from build123d import *

# Parameters (mm, degrees)
BOSS_EXTRUDE1_DEPTH      = 8.2
BOSS_EXTRUDE1_DEPTH_BACK = 8.2
SKETCH2_W                = 10
SKETCH2_H                = 42
CUT_EXTRUDE1_DEPTH       = 25.662522174
CUT_EXTRUDE1_DEPTH_BACK  = 25.662522174
SKETCH4_R                = 1
SKETCH4_W                = 13.4
SKETCH4_H                = 24
CIRPATTERN1_COUNT        = 4
BOSS_EXTRUDE2_DEPTH      = 8
BOSS_EXTRUDE3_DEPTH      = 8
BOSS_EXTRUDE4_DEPTH      = 6
BOSS_EXTRUDE5_START      = 6
SKETCH23_R               = 37.2
BOSS_EXTRUDE5_DEPTH      = 6


with BuildPart() as part:
    # Sketch2 → Boss-Extrude1 (new, two sides: drawn at the far end of the back side and taken through both)
    with BuildSketch(Plane(origin=(0, 0, 0), x_dir=(0, 0, -1), z_dir=(1, 0, 0)).offset(-BOSS_EXTRUDE1_DEPTH_BACK)):
        with Locations((-22, 0)):
            Rectangle(SKETCH2_W, SKETCH2_H)
    extrude(amount=BOSS_EXTRUDE1_DEPTH + BOSS_EXTRUDE1_DEPTH_BACK)

    # Sketch4 → Cut-Extrude1 (cut, two sides: drawn at the far end of the back side and taken through both)
    with BuildSketch(Plane.XY.offset(27).offset(-CUT_EXTRUDE1_DEPTH_BACK)):
        with Locations((-3, 14.95)):
            Circle(SKETCH4_R)
        with Locations((2.95, 14.95)):
            Circle(SKETCH4_R)
        with Locations((-3, -14.95)):
            Circle(SKETCH4_R)
        with Locations((2.95, -14.95)):
            Circle(SKETCH4_R)
        with Locations((1.5, 0)):
            Rectangle(SKETCH4_W, SKETCH4_H)
    extrude(amount=CUT_EXTRUDE1_DEPTH + CUT_EXTRUDE1_DEPTH_BACK, mode=Mode.SUBTRACT)


with BuildPart() as cirpattern1_1:
    # CirPattern1: pattern copy
    add(part.part.rotate(Axis((0, 0, 0), (0, 1, 0)), 1 * 360 / CIRPATTERN1_COUNT))


with BuildPart() as cirpattern1_2:
    # CirPattern1: pattern copy
    add(part.part.rotate(Axis((0, 0, 0), (0, 1, 0)), 2 * 360 / CIRPATTERN1_COUNT))


with BuildPart() as cirpattern1_3:
    # CirPattern1: pattern copy
    add(part.part.rotate(Axis((0, 0, 0), (0, 1, 0)), 3 * 360 / CIRPATTERN1_COUNT))


with BuildPart() as part_1:
    add(part.part)

    add(cirpattern1_1.part)  # Boss-Extrude2 merges CirPattern1_1

    add(cirpattern1_2.part)  # Boss-Extrude2 merges CirPattern1_2

    add(cirpattern1_3.part)  # Boss-Extrude2 merges CirPattern1_3
    # Sketch20 → Boss-Extrude2 (add)
    with BuildSketch(Plane(origin=(0, 21, 0), x_dir=(1, 0, 0), z_dir=(0, 1, 0))):
        Polygon((-17, 8.2), (-8.2, 17), (-8.2, 27), (-27, 8.2), align=None)
        Polygon((-17, -8.2), (-8.2, -17), (-8.2, -27), (-27, -8.2), align=None)
        Polygon((8.2, -17), (17, -8.2), (27, -8.2), (8.2, -27), align=None)
        Polygon((8.2, 17), (17, 8.2), (27, 8.2), (8.2, 27), align=None)
    extrude(amount=-BOSS_EXTRUDE2_DEPTH)

    # Sketch21 → Boss-Extrude3 (add)
    with BuildSketch(Plane.XZ.offset(21)):
        Polygon((-17, 8.2), (-8.2, 17), (-8.2, 27), (-27, 8.2), align=None)
        Polygon((17, -8.2), (8.2, -17), (8.2, -27), (27, -8.2), align=None)
        Polygon((-8.2, -17), (-17, -8.2), (-27, -8.2), (-8.2, -27), align=None)
        Polygon((8.2, 17), (17, 8.2), (27, 8.2), (8.2, 27), align=None)
    extrude(amount=-BOSS_EXTRUDE3_DEPTH)

    # Sketch22 → Boss-Extrude4 (add)
    with BuildSketch(Plane.XZ.offset(21)):
        with BuildLine():
            ThreePointArc((-15.663157895, 33.741746913), (-26.30437226, 26.30437226), (-33.741746913, 15.663157895))
            Line((-33.741746913, 15.663157895), (-33.274371034, 15.663157895))
            Line((-33.274371034, 15.663157895), (-33.274371034, -15.663157895))
            Line((-33.274371034, -15.663157895), (-33.741746913, -15.663157895))
            ThreePointArc((-33.741746913, -15.663157895), (-26.30437226, -26.30437226), (-15.663157895, -33.741746913))
            Line((-15.663157895, -33.741746913), (-15.663157895, -33.274371034))
            Line((-15.663157895, -33.274371034), (15.663157895, -33.274371034))
            Line((15.663157895, -33.274371034), (15.663157895, -33.741746913))
            ThreePointArc((15.663157895, -33.741746913), (26.30437226, -26.30437226), (33.741746913, -15.663157895))
            Line((33.741746913, -15.663157895), (33.274371034, -15.663157895))
            Line((33.274371034, -15.663157895), (33.274371034, 15.663157895))
            Line((33.274371034, 15.663157895), (33.741746913, 15.663157895))
            ThreePointArc((33.741746913, 15.663157895), (26.30437226, 26.30437226), (15.663157895, 33.741746913))
            Line((15.663157895, 33.741746913), (15.663157895, 33.274371034))
            Line((15.663157895, 33.274371034), (-15.663157895, 33.274371034))
            Line((-15.663157895, 33.274371034), (-15.663157895, 33.741746913))
        make_face()
        Polygon((17, -8.2), (8.2, -17), (-8.2, -17), (-17, -8.2), (-17, 8.2), (-8.2, 17), (8.2, 17), (17, 8.2), align=None, mode=Mode.SUBTRACT)
    extrude(amount=BOSS_EXTRUDE4_DEPTH)

    # Sketch23 → Boss-Extrude5 (add)
    with BuildSketch(Plane(origin=(0, 21, 0), x_dir=(1, 0, 0), z_dir=(0, 1, 0)).offset(BOSS_EXTRUDE5_START)):
        with Locations(Location((0, 0, 0), (0, 0, 270))):
            Circle(SKETCH23_R)
        Polygon((-17, 8.2), (-8.2, 17), (8.2, 17), (17, 8.2), (17, -8.2), (8.2, -17), (-8.2, -17), (-17, -8.2), align=None, mode=Mode.SUBTRACT)
    extrude(amount=-BOSS_EXTRUDE5_DEPTH)


solid = part_1.part
Here's how the part is built. I have some questions about the finished solid (model axes, mm). A direction names the side the tool comes from. Give positions to 0.01 mm unless a question says otherwise; leave off trailing zeros. Order: outer loops, then holes, each group sorted by start corner. A loop starts at its lowest first (then second) coordinate and runs counter-clockwise, first axis right, second up. Notation, with made-up numbers: M 62.25,48.5 L 80.25,48.5 A21 cw 80.25,72.5 Z; hole C 19,-30.75 d11. An arc over 180 degrees is marked long. Answer as a JSON object with one key per item and string values. Group by question number.
1) Suppose I cut it at A-A, the plane y = 11. Write out the boundary of the cut face in (x, z), plus the area to 3 significant figures.
2) On a 3-axis mill with a long thin cutter (end or side, diameter ignored), from which of +Z, -Z, +X, -X, +Y, -Y can I reach the whole of each face in a straight line? I mean faces 1 (the flat face through (1, 12, 22)), 2 (the flat face through (-27, 0, -6)), 3 (the flat face through (27, 0, 6)), 4 (the flat face through (6, 0, -27)). Say none if no direction works.
3) Suppose I cut it at C-C, the plane x = -31. Write out the boundary of the cut face in (y, z), plus the area to 3 significant figures.
4) Suppose I cut it at B-B, the plane z = 0. Write out the boundary of the cut face in (x, y).
5) I'm going to push flat-ended pins straight in: pin 1 Ø13 at (y, z) = (9.5, -2) entering from -X; pin 2 Ø10 at (y, z) = (-18, 21) entering from -X; pin 3 Ø12 at (y, z) = (-20, 14) entering from +X. Where does each tip first touch, or does it pass through?
6) We'd pull the mould along Z, two halves only. Please class faces 5 (the flat face through (-17.5, -17.1, 17.7)), 6 (the cylindrical face through (21.93, 13.974, -2.733)), 7 (the flat face through (-15, -13, 16)): pulls with the +Z half, pulls with the -Z half, needs draft (parallel to the pull), parting line crosses it, or undercut.
7) Suppose I cut it at D-D, the plane x = -12.5. Write out the boundary of the cut face in (y, z).
8) Please list where these lines run through material, in increasing order: L1, parallel to Y at x = -19.75, z = -3; L2, parallel to Y at x = 15.5, z = -13; L3, parallel to Y at x = -5.5, z = -28. Write a range as [from, to].
Results found:
{
 "1": {"outline": "M -27,-8.2 L -17,-8.2 L -17,-5.2 L -27,-5.2 Z; M -8.2,17 L -5.2,17 L -5.2,27 L -8.2,27 Z; M 5.2,-27 L 8.2,-27 L 8.2,-17 L 5.2,-17 Z; M 17,5.2 L 27,5.2 L 27,8.2 L 17,8.2 Z", "area": "120 mm²"},
 "2": {"face 1": "+Z, +X", "face 2": "+Z, -Z, -X", "face 3": "+Z, -Z, +X", "face 4": "-Z, +X, -X"},
 "3": {"outline": "M -27,-20.56 L -21,-20.56 L -21,20.56 L -27,20.56 Z; M 21,-20.56 L 27,-20.56 L 27,20.56 L 21,20.56 Z", "area": "494 mm²"},
 "4": {"outline": "M -37.2,21 L -27,21 L -27,12 L -17,12 L -17,27 L -37.2,27 Z; M -33.27,-27 L -17,-27 L -17,-12 L -27,-12 L -27,-21 L -33.27,-21 Z; M 17,-27 L 33.27,-27 L 33.27,-21 L 27,-21 L 27,-12 L 17,-12 Z; M 17,12 L 27,12 L 27,21 L 37.2,21 L 37.2,27 L 17,27 Z"},
 "5": {"pin 1": "x = -27", "pin 2": "x = -33.09", "pin 3": "x = 33.74"},
 "6": {"face 5": "pulls with the +Z half", "face 6": "undercut", "face 7": "needs draft"},
 "7": {"outline": "M -27,-33.27 L -21,-33.27 L -21,-22.7 L -13,-22.7 L -13,-12.7 L -27,-12.7 Z; M -27,12.7 L -13,12.7 L -13,22.7 L -21,22.7 L -21,33.27 L -27,33.27 Z; M 13,-22.7 L 21,-22.7 L 21,-35.04 L 27,-35.04 L 27,-12.7 L 13,-12.7 Z; M 13,12.7 L 27,12.7 L 27,35.04 L 21,35.04 L 21,22.7 L 13,22.7 Z"},
 "8": {"L1": "[-27, -15.95], [-13.95, -12], [12, 13.95], [15.95, 27]", "L2": "[-27, -13], [13, 27]", "L3": "[-27, -21], [21, 27]"}
}
